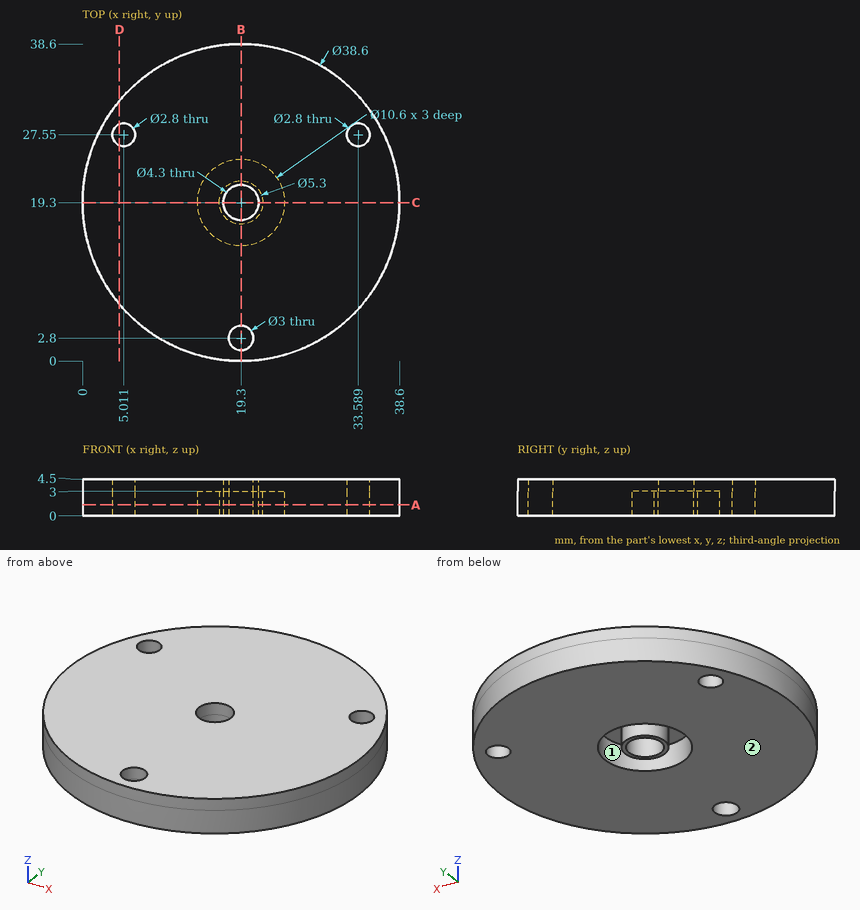
Geometry check sheet. Reference: drawing and pictorial views, mm from the part's lowest x, y, z. Coordinates: 2 decimals unless noted, no trailing zeros. Write each loop counter-clockwise with the first axis right and the second up, starting at its lowest first coordinate (ties: lowest second). Pieces come first, ordered by that corner, then holes. Notation, with made-up numbers: (-6, 74) -> (-1, 74) arc R12 ccw to (-1, 86) -> close; hole circle Ø10 at (43.25, -2.75). An arc over 180 degrees is marked (long way). Use a Markdown table: item, result.
1. Scan lines: line 1 along Y through (x, z) = (19.3, 3.8); line 2 along X through (y, z) = (19.3, 4); line 3 along X through (y, z) = (27.55, 1.5). Record each from-to range of solid material in increasing order.
Reported:
| item | result |
|---|---|
| line 1 | y = 0 to 1.3, 4.3 to 17.15, 21.45 to 38.6 |
| line 2 | x = 0 to 17.15, 21.45 to 38.6 |
| line 3 | x = 1.85 to 3.61, 6.41 to 32.19, 34.99 to 36.75 |
2. Sectioned sample at C-C (y = 19.3). Enter the section's corners in (x, z).
Reported:
| item | result |
|---|---|
| outline | (0, 0) -> (14, 0) -> (14, 3) -> (16.65, 3) -> (16.65, 0) -> (17.15, 0) -> (17.15, 4.5) -> (0, 4.5) -> close; (21.45, 0) -> (21.95, 0) -> (21.95, 3) -> (24.6, 3) -> (24.6, 0) -> (38.6, 0) -> (38.6, 4.5) -> (21.45, 4.5) -> close |
3. Sectioned sample at A-A (z = 1.35). Enter the section's corners in (x, y).
Reported:
| item | result |
|---|---|
| outline | circle Ø38.6 at (19.3, 19.3); circle Ø5.3 at (19.3, 19.3); hole circle Ø2.8 at (5.01, 27.55); hole circle Ø10.6 at (19.3, 19.3); hole circle Ø4.3 at (19.3, 19.3); hole circle Ø3 at (19.3, 2.8); hole circle Ø2.8 at (33.59, 27.55) |
4. Release check for a two-part mould opening along X. For the marked faces 1 and 2 record: pulls with the +X half, pulls with the -X half, needs draft (parallel to the pull), parting line crosses it, or undercut.
Reported:
| item | result |
|---|---|
| face 1 | undercut |
| face 2 | needs draft |
5. Sectioned sample at D-D (x = 4.5). Enter the section's corners in (y, z).
Reported:
| item | result |
|---|---|
| outline | (6.91, 0) -> (26.25, 0) -> (26.25, 4.5) -> (6.91, 4.5) -> close; (28.85, 0) -> (31.69, 0) -> (31.69, 4.5) -> (28.85, 4.5) -> close |
6. Sectioned sample at B-B (x = 19.3). Enter the section's corners in (y, z).
Reported:
| item | result |
|---|---|
| outline | (0, 0) -> (1.3, 0) -> (1.3, 4.5) -> (0, 4.5) -> close; (4.3, 0) -> (14, 0) -> (14, 3) -> (16.65, 3) -> (16.65, 0) -> (17.15, 0) -> (17.15, 4.5) -> (4.3, 4.5) -> close; (21.45, 0) -> (21.95, 0) -> (21.95, 3) -> (24.6, 3) -> (24.6, 0) -> (38.6, 0) -> (38.6, 4.5) -> (21.45, 4.5) -> close |
